Design review of the part built by this model. Coordinates are the model's own, in mm. Face numbers are marked on the shaded views. A direction names the side the tool comes from. Coordinates: 2 decimals unless noted, no trailing zeros. Write each loop counter-clockwise with the first axis right and the second up, starting at its lowest first coordinate (ties: lowest second). Pieces come first, ordered by that corner, then holes. Notation, with made-up numbers: M 8.25,89.25 L 55.25,89.25 A33 ccw 55.25,128.25 Z; hole C 59.5,66 d1. An arc over 180 degrees is marked long. Write item = value, one per line.
```python
from build123d import *

# Parameters (mm, degrees)
BOSS_EXTRUDE1_DEPTH      = 1
BOSS_EXTRUDE1_DEPTH_BACK = 3
FILLET1_R                = 0.1


with BuildPart() as part:
    # Sketch3 → Boss-Extrude1 (new, two sides: drawn at the far end of the back side and taken through both)
    with BuildSketch(Plane.YZ.offset(-BOSS_EXTRUDE1_DEPTH_BACK)):
        with BuildLine():
            Line((-4, 5.4), (-1.56416825, 5.4))
            ThreePointArc((-1.56416825, 5.4), (-1.195386471, 5.645080666), (-1.278511113, 6.08))
            ThreePointArc((-1.278511113, 6.08), (-1.403198074, 6.732379001), (-0.850025407, 7.1))
            Line((-0.850025407, 7.1), (0.850025407, 7.1))
            ThreePointArc((0.850025407, 7.1), (1.403198074, 6.732379001), (1.278511113, 6.08))
            ThreePointArc((1.278511113, 6.08), (1.195386471, 5.645080666), (1.56416825, 5.4))
            Line((1.56416825, 5.4), (4, 5.4))
            ThreePointArc((4, 5.4), (4.322991043, 5.564040711), (4.381063684, 5.92161607))
            Line((4.381063684, 5.92161607), (2.881063684, 10.62161607))
            ThreePointArc((2.881063684, 10.62161607), (2.735959289, 10.822991043), (2.5, 10.9))
            Line((2.5, 10.9), (-2.5, 10.9))
            ThreePointArc((-2.5, 10.9), (-2.735959289, 10.822991043), (-2.881063684, 10.62161607))
            Line((-2.881063684, 10.62161607), (-4.381063684, 5.92161607))
            ThreePointArc((-4.381063684, 5.92161607), (-4.322991043, 5.564040711), (-4, 5.4))
        make_face()
    extrude(amount=BOSS_EXTRUDE1_DEPTH + BOSS_EXTRUDE1_DEPTH_BACK)

    # Fillet1
    fillet1_edges = [part.edges().sort_by_distance(p)[0] for p in [
        (-3, -1.195386471, 5.645080666),
        (-3, -1.403198074, 6.732379001),
        (-3, 0, 7.1),
        (-3, 1.403198074, 6.732379001),
        (-3, 1.195386471, 5.645080666),
        (-3, 2.782084125, 5.4),
        (-3, 4.322991043, 5.564040711),
        (1, -4.322991043, 5.564040711),
        (1, -2.782084125, 5.4),
        (1, -1.195386471, 5.645080666),
        (1, -1.403198074, 6.732379001),
        (-3, 3.631063684, 8.27161607),
        (1, 0, 7.1),
        (1, 1.403198074, 6.732379001),
        (1, 1.195386471, 5.645080666),
        (1, 2.782084125, 5.4),
        (1, 4.322991043, 5.564040711),
        (1, 3.631063684, 8.27161607),
        (1, 2.735959289, 10.822991043),
        (1, 0, 10.9),
        (1, -2.735959289, 10.822991043),
        (1, -3.631063684, 8.27161607),
        (-3, 2.735959289, 10.822991043),
        (-3, 0, 10.9),
        (-3, -4.322991043, 5.564040711),
        (-3, -2.735959289, 10.822991043),
        (-3, -3.631063684, 8.27161607),
        (-3, -2.782084125, 5.4),
    ]]
    fillet(fillet1_edges, radius=FILLET1_R)


solid = part.part
```
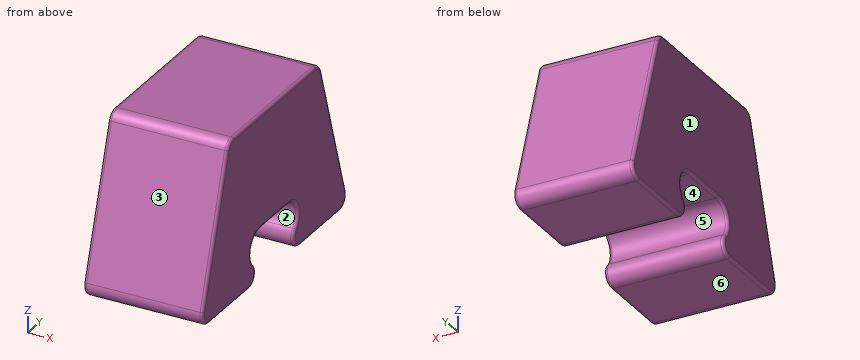
Q1. Machinability: for the marked faces 4, 5 and 6, which of the approach directions +Z, -Z, +X, -X, +Y, -Y give a long, thin tool a straight path to every point of the face, cutting with its end or side? Answer none if there is none.
Check result:
face_4 = -Z, +X, -X
face_5 = +X, -X
face_6 = -Z, +X, -X, +Y, -Y
Q2. The part is to be moulded in two halves that separate along Y. For the marked faces 1, 2 and 3, say which applies: +Y half, -Y half, draft (parallel to the pull), parting line (faces both ways), or undercut.
Check result:
face_1 = draft
face_2 = undercut
face_3 = -Y half
Q3. Consider section A-A, the plane y = -0.25. State the section outline as (x, z) points.
Check result:
outline = M -3,7.2 A0.1 ccw -2.9,7.1 L 0.9,7.1 A0.1 ccw 1,7.2 L 1,10.8 A0.1 ccw 0.9,10.9 L -2.9,10.9 A0.1 ccw -3,10.8 Z
Q4. Consider section B-B, the plane x = -0.9. State the section outline as (y, z) points.
Check result:
outline = M -4.38,5.92 A0.4 ccw -4,5.4 L -1.56,5.4 A0.4 ccw -1.28,6.08 A0.6 cw -0.85,7.1 L 0.85,7.1 A0.6 cw 1.28,6.08 A0.4 ccw 1.56,5.4 L 4,5.4 A0.4 ccw 4.38,5.92 L 2.88,10.62 A0.4 ccw 2.5,10.9 L -2.5,10.9 A0.4 ccw -2.88,10.62 Z
Q5. Wall thickness on line 1 (Z direction, x = -1.1, y = -0.5); line 2 (Y direction, x = -1.15, z = 6.9); line 3 (Y direction, x = -0.7, z = 6.05): over which ranges is each line inside the solid? List them lowest first.
Check result:
line_1 = 7.1 to 10.9
line_2 = -4.07 to -1.3, 1.3 to 4.07
line_3 = -4.34 to -1.25, 1.25 to 4.34
Q6. For P1, Ø2, axis at x = -1.5, y = 0.5, coming from the -Z side, flat-tipped, find the tip position at first contact; note if it passes through.
Check result:
P1 = 5.41
